Design review of the part built by this model. Coordinates are the model's own, in mm. Face numbers are marked on the shaded views. A direction names the side the tool comes from. Round coordinates to 2 decimals unless told otherwise and drop trailing zeros. Order: outer loops, then holes, each group sorted by start corner. A loop starts at its lowest first (then second) coordinate and runs counter-clockwise, first axis right, second up.
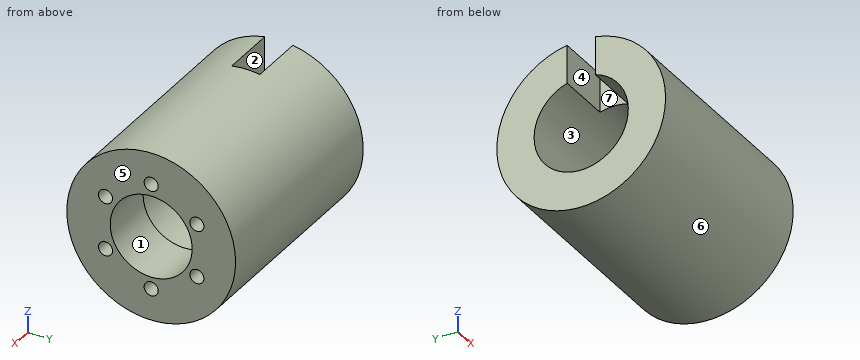
from build123d import *

# Parameters (mm, degrees)
SKETCH1_W          = 25.4
SKETCH1_H          = 5.3975
SKETCH2_R          = 3.175
SKETCH2_R_2        = 18.5
CUT_EXTRUDE1_DEPTH = 25.4
CIRPATTERN1_COUNT  = 6
SKETCH3_W          = 25.4
SKETCH3_H          = 12.7
CUT_EXTRUDE2_DEPTH = 39.1


with BuildPart() as part:
    # Sketch1 → Revolve1 (revolve)
    with BuildSketch(Plane.XY):
        Polygon((-49.2125, 38.1), (-49.2125, 21.2725), (23.8125, 21.2725), (49.2125, 21.2725), (49.2125, 38.1), (42.8625, 38.1), align=None)
        with Locations((36.5125, 18.57375)):
            Rectangle(SKETCH1_W, SKETCH1_H)
    revolve(axis=Axis((-49.2125, 0, 0), (1, 0, 0)))

    # Sketch2 → Cut-Extrude1 (cut)
    with BuildSketch(Plane(origin=(49.2125, 0, 0), x_dir=(0, 0, -1), z_dir=(1, 0, 0))):
        with Locations((-11.90625, -20.622229928)):
            Circle(SKETCH2_R)
        with Locations((11.90625, -20.622229928)):
            Circle(SKETCH2_R)
        with Locations((23.8125, 0)):
            Circle(SKETCH2_R)
        with Locations((11.90625, 20.622229928)):
            Circle(SKETCH2_R)
        with Locations((-11.90625, 20.622229928)):
            Circle(SKETCH2_R)
        Circle(SKETCH2_R_2)
    cut_extrude1 = extrude(amount=-CUT_EXTRUDE1_DEPTH, mode=Mode.SUBTRACT)

    # CirPattern1: Cut-Extrude1 ×6 about axis
    cirpattern1_axis = Axis((-49.2125, 0, 0), (-1, 0, 0))
    for i in range(1, CIRPATTERN1_COUNT):
        add(cut_extrude1.rotate(cirpattern1_axis, i * 360 / CIRPATTERN1_COUNT), mode=Mode.SUBTRACT)

    # Sketch3 → Cut-Extrude2 (cut, through all)
    with BuildSketch(Plane.XY):
        with Locations((-36.5125, 0)):
            Rectangle(SKETCH3_W, SKETCH3_H)
    extrude(amount=CUT_EXTRUDE2_DEPTH, mode=Mode.SUBTRACT)


solid = part.part
1) Take a section at C-C on x = -14. Give the boundary of the cut face in (y, z) (1 decimal), plus the area to 3 significant figures.
Results:
outline: circle Ø76.2 at (0, 0); hole circle Ø42.5 at (0, 0)
area: 3,140 mm2
2) Take a section at B-B on y = 12. Give the boundary of the cut face in (x, z).
Results:
outline: (-49.21, -36.16) - (49.21, -36.16) - (49.21, -14.08) - (23.81, -14.08) - (23.81, -17.56) - (-49.21, -17.56) - close; (-49.21, 17.56) - (23.81, 17.56) - (23.81, 14.08) - (49.21, 14.08) - (49.21, 36.16) - (-49.21, 36.16) - close
3) The part is to be moulded in two halves that separate along Y. For the marked faces 4, 5, 6 and 7, say which applies: released by +Y, released by -Y, zero draft, split by the parting line, or undercut.
Results:
face 4: undercut
face 5: zero draft
face 6: split by the parting line
face 7: undercut
4) Clearance check with flat-ended pins moving along their axes: P1, Ø3, axis at y = 22, z = -12.5, coming from the +X side; P2, Ø10, axis at x = -19.5, z = 3.5, coming from the -Y side; P3, Ø1.5, axis at y = 18, z = -4, coming from the -X side; P4, Ø2, axis at x = 39, y = -21.5, coming from the +Z side. State where each tip first meets the part, or that it passes through.
Results:
P1: stops at x = 23.81
P2: stops at y = -38.1
P3: stops at x = 23.81
P4: stops at z = 32.11
5) Take a section at A-A on y = 0. Give the boundary of the cut face in (x, z).
Results:
outline: (-49.21, -38.1) - (49.21, -38.1) - (49.21, -26.99) - (23.81, -26.99) - (23.81, -21.27) - (-49.21, -21.27) - close; (-23.81, 21.27) - (23.81, 21.27) - (23.81, 26.99) - (49.21, 26.99) - (49.21, 38.1) - (-23.81, 38.1) - close; (23.81, -20.64) - (49.21, -20.64) - (49.21, -18.5) - (23.81, -18.5) - close; (23.81, 18.5) - (49.21, 18.5) - (49.21, 20.64) - (23.81, 20.64) - close
6) For the marked faces 1, 2 and 3, list the 3-axis set-ups (+Z, -Z, +X, -X, +Y, -Y) from which the entire face can be reached by the end or side of a thin tool; tool diameter is ignored.
Results:
face 1: +X, -X
face 2: +Z, -X
face 3: -X
7) To check wall thickness, follow line 1 along Z through (x, y) = (33, 0); line 2 along Z through (x, y) = (26.5, -20); line 3 along Z through (x, y) = (-5, -9). State the ranges of each line that lie inside material, in increasing order.
Results:
line 1: z = -38.1 to -26.99, -20.64 to -18.5, 18.5 to 20.64, 26.99 to 38.1
line 2: z = -32.43 to -15.02, -8.79 to 8.79, 15.02 to 32.43
line 3: z = -37.02 to -19.27, 19.27 to 37.02
8) Take a section at D-D on z = 17. Give the boundary of the cut face in (x, y).
Results:
outline: (-49.21, -34.1) - (49.21, -34.1) - (49.21, -7.3) - (23.81, -7.3) - (23.81, -12.79) - (-49.21, -12.79) - close; (-49.21, 12.79) - (23.81, 12.79) - (23.81, 7.3) - (49.21, 7.3) - (49.21, 34.1) - (-49.21, 34.1) - close
